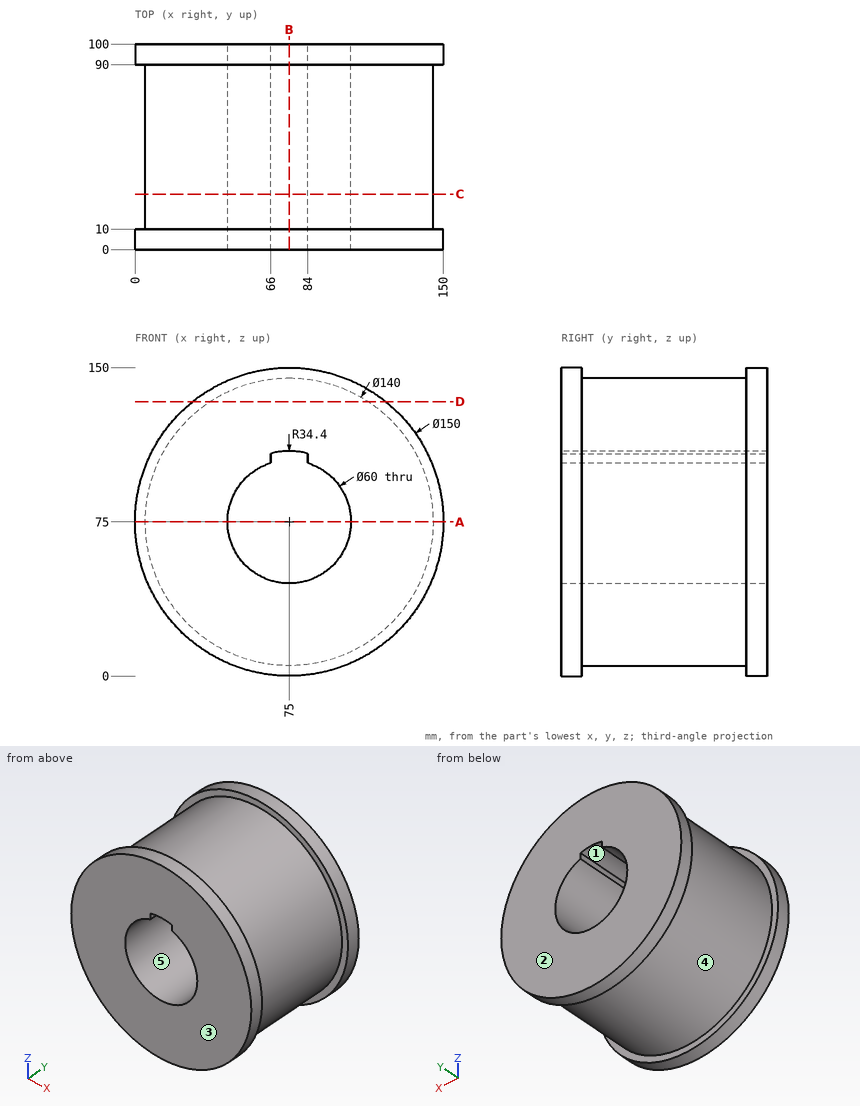
The figure shows three views and two pictorial views of one solid part (mm, origin at its lowest corner). Answer the questions. A direction names the side the tool comes from. Give positions to 0.01 mm unless a question says otherwise; leave off trailing zeros. Write each loop counter-clockwise with the first axis right and the second up, starting at its lowest first coordinate (ties: lowest second). Pieces come first, ordered by that corner, then holes. Notation, with made-up numbers: M -28.75,-37 L 25.25,-37 A8 ccw 25.25,-24 Z; hole C 75.25,81.5 d1. An arc over 180 degrees is marked long. Write each question's results on one line, items separated by ' | '.
Q1. For a pull along X with two mould halves and no side action, classify the marked faces 3, 4 and 5 as released by +X, released by -X, zero draft, split by the parting line, or undercut.
Output values:
face 3: zero draft | face 4: split by the parting line | face 5: undercut
Q2. Section A-A, the plane z = 75 is taken. Write down the section's boundary in (x, y), then the cut area to 3 significant figures.
Output values:
outline: M 0,0 L 45,0 L 45,100 L 0,100 L 0,90 L 5,90 L 5,10 L 0,10 Z; M 105,0 L 150,0 L 150,10 L 145,10 L 145,90 L 150,90 L 150,100 L 105,100 Z | area: 8,200 mm2
Q3. Flat-ended cylindrical pins translate along their axes: P1, Ø5, axis at y = 44, z = 20, coming from the +X side; P2, Ø10, axis at y = 76, z = 34, coming from the +X side; P3, Ø8, axis at y = 15.5, z = 39, coming from the -X side. Find the tip coordinate at first contact, or state that the pin passes through.
Output values:
P1: x = 121.3 | P2: x = 135.03 | P3: x = 12.74
Q4. Consider L1, parallel to X at y = 63, z = 75; L2, parallel to X at y = 86, z = 92; L3, parallel to Y at x = 12, z = 44. Determine where each line is inside the solid, lowest interval first. Write a range as from..to.
Output values:
L1: 5..45, 105..145 | L2: 7.1..50.28, 99.72..142.9 | L3: 0..10, 90..100
Q5. Section B-B, the plane x = 75 is taken. Write down the section's boundary in (y, z).
Output values:
outline: M 0,0 L 10,0 L 10,5 L 90,5 L 90,0 L 100,0 L 100,45 L 0,45 Z; M 0,109.4 L 100,109.4 L 100,150 L 90,150 L 90,145 L 10,145 L 10,150 L 0,150 Z
Q6. Section C-C, the plane y = 27 is taken. Write down the section's boundary in (x, z), then the cut area to 3 significant figures.
Output values:
outline: C 75,75 d140; hole M 66,103.62 A30 ccw long 84,103.62 L 84,108.2 A34.4 ccw 66,108.2 Z | area: 12,500 mm2
Q7. A tool of negligible diameter and unlimited length cuts with its end or side. For the marked faces 1 and 2, from which of +Z, -Z, +X, -X, +Y, -Y can it reach the whole face along a straight path? Write none if from no direction.
Output values:
face 1: +Y, -Y | face 2: +Z, -Z, +X, -X, +Y
Q8. Section D-D, the plane z = 133.5 is taken. Write down the section's boundary in (x, y), then the cut area to 3 significant figures.
Output values:
outline: M 28.07,0 L 121.93,0 L 121.93,10 L 113.44,10 L 113.44,90 L 121.93,90 L 121.93,100 L 28.07,100 L 28.07,90 L 36.56,90 L 36.56,10 L 28.07,10 Z | area: 8,030 mm2
